```python
from build123d import *

# Parameters (mm, degrees)
SKETCH_W     = 232
SKETCH_H     = 75
PAD_DEPTH    = 1
SKETCH001_R  = 2.5
POCKET_DEPTH = 5


with BuildPart() as part:
    # Sketch → Pad (new body)
    with BuildSketch(Plane.XY):
        Rectangle(SKETCH_W, SKETCH_H)
    extrude(amount=PAD_DEPTH)

    # Sketch001 (on Face6 of Pad) → Pocket (cut)
    with BuildSketch(Plane.XY.offset(1)):
        with Locations((-68.1, 3.4)):
            Circle(SKETCH001_R)
        with Locations((71.1, 3.4)):
            Circle(SKETCH001_R)
        Polygon((-5.320624, -16.015108), (-5.320624, 17.20542), (-10.320624, 17.20542), (0, 26.156277), (10.320624, 17.20542), (5.320624, 17.20542), (5.320624, -16.015108), align=None)
    extrude(amount=-POCKET_DEPTH, mode=Mode.SUBTRACT)


solid = part.part
```
Could you check a few things on this model? Use its own coordinates, in mm. Coordinates: 2 decimals unless noted, no trailing zeros. Loops run counter-clockwise (first coordinate to the right, second up) from the corner with the lowest first, then second, coordinate; pieces in that order, holes last. Notation, with made-up numbers: M 65,17.25 L 118,17.25 A25 cw 118,56.25 Z; hole C 82,56 d9. An arc over 180 degrees is marked long. Put each result on its own line as item: value. Start each with the question number.
(1) Suppose I cut it at A-A on x = -68.1. Please give me the cut outline in (y, z).
(2) Suppose I cut it at C-C on z = 0.4. Please give me the cut outline in (x, y), then the cut area to 3 significant figures.
(3) Will this pin go through, and if not, where does the flat tip stop? P1, Ø6, axis at x = 71.1, y = 3.4, coming from the -Z side.
(4) Suppose I cut it at B-B on y = -3.5. Please give me the cut outline in (x, z), then the cut area to 3 significant figures.
(5) I need wall thicknesses on line 1 (Y direction, x = -68, z = 0.85); line 2 (X direction, y = -5.5, z = 0.45); line 3 (X direction, y = 5.5, z = 0.7). Which ranges of each line are inside material? Lowest first, please. Write a range as from..to.
(6) Thinking about a two-plate mould opening in Y: for faces 1 (the face through (-70.6, 3.5, 0.5)), 2 (the face through (-2, -24, 0)), which applies, pulls with the +Y half, pulls with the -Y half, needs draft (parallel to the pull), parting line crosses it, or undercut?
Solutions:
1. outline: M -37.5,0 L 0.9,0 L 0.9,1 L -37.5,1 Z; M 5.9,0 L 37.5,0 L 37.5,1 L 5.9,1 Z
2. outline: M -116,-37.5 L 116,-37.5 L 116,37.5 L -116,37.5 Z; hole C -68.1,3.4 d5; hole M -10.32,17.21 L -5.32,17.21 L -5.32,-16.02 L 5.32,-16.02 L 5.32,17.21 L 10.32,17.21 L 0,26.16 Z; hole C 71.1,3.4 d5
2. area: 16,900 mm2
3. P1: stops at z = 0
4. outline: M -116,0 L -5.32,0 L -5.32,1 L -116,1 Z; M 5.32,0 L 116,0 L 116,1 L 5.32,1 Z
4. area: 221 mm2
5. line 1: y = -37.5..0.9, 5.9..37.5
5. line 2: x = -116..-5.32, 5.32..116
5. line 3: x = -116..-69.46, -66.74..-5.32, 5.32..69.74, 72.46..116
6. face 1: undercut
6. face 2: needs draft
